Geometry: final body of the model. Coordinates: model frame, mm. Give positions to 0.01 mm unless a question says otherwise; leave off trailing zeros. Write each loop counter-clockwise with the first axis right and the second up, starting at its lowest first coordinate (ties: lowest second). Pieces come first, ordered by that corner, then holes.
from build123d import *

# Parameters (mm, degrees)
SKETCH1_W               = 127
SKETCH1_H               = 152.4
BOSS_EXTRUDE1_DEPTH     = 1.6
CHAMFER1_SIZE           = 5
CHAMFER2_SIZE           = 1.27
SKETCH4_OUTSIDE_W       = 168.678
SKETCH4_OUTSIDE_H       = 194.078
SKETCH4_OUTSIDE_W_2     = 146.645454771
SKETCH4_OUTSIDE_H_2     = 144.4
CUT_EXTRUDE3_DEPTH      = 0.0001
CUT_EXTRUDE4_DEPTH      = 100.203074549
CUT_EXTRUDE4_DEPTH_BACK = 100.203074549
SKETCH7_W               = 10
SKETCH7_H               = 16
CUT_EXTRUDE7_DEPTH      = 10
CUT_EXTRUDE8_REACH      = 101.203
SKETCH9_R               = 1.75


with BuildPart() as part:
    # Sketch1 → Boss-Extrude1 (new body)
    with BuildSketch(Plane(origin=(0, 0, 0), x_dir=(1, 0, 0), z_dir=(0, 1, 0))):
        Rectangle(SKETCH1_W, SKETCH1_H)
    extrude(amount=BOSS_EXTRUDE1_DEPTH)

    # Chamfer1
    chamfer1_edges = [part.edges().sort_by_distance(p)[0] for p in [
        (-63.5, 0.8, 76.2),
        (-63.5, 0.8, -76.2),
    ]]
    chamfer(chamfer1_edges, length=CHAMFER1_SIZE)

    # Chamfer2
    chamfer2_edges = [part.edges().sort_by_distance(p)[0] for p in [
        (63.5, 0.8, 76.2),
        (63.5, 0.8, -76.2),
    ]]
    chamfer(chamfer2_edges, length=CHAMFER2_SIZE)

    # Sketch4 outside → Cut-Extrude3 (cut)
    with BuildSketch(Plane(origin=(0, 1.6, 0), x_dir=(-1, 0, 0), z_dir=(0, 1, 0))):
        Rectangle(SKETCH4_OUTSIDE_W, SKETCH4_OUTSIDE_H)
        with Locations((0.842207065, 0)):
            Rectangle(SKETCH4_OUTSIDE_W_2, SKETCH4_OUTSIDE_H_2, mode=Mode.SUBTRACT)
    extrude(amount=-CUT_EXTRUDE3_DEPTH, mode=Mode.SUBTRACT)

    # Sketch5 → Cut-Extrude4 (cut, two sides: drawn at the far end of the back side and taken through both)
    with BuildSketch(Plane(origin=(0, 1.6, 0), x_dir=(1, 0, 0), z_dir=(0, 1, 0)).offset(-CUT_EXTRUDE4_DEPTH_BACK)):
        Polygon((-8.552407118, -467.338817365), (-53, -76.2), (-63.5, 16.2), (-107.947592882, 407.338817365), (-890.225227612, 318.4436316), (-790.830041847, -556.23400313), align=None)
    extrude(amount=CUT_EXTRUDE4_DEPTH + CUT_EXTRUDE4_DEPTH_BACK, mode=Mode.SUBTRACT)

    # Sketch7 → Cut-Extrude7 (cut)
    with BuildSketch(Plane(origin=(0, 1.6, 0), x_dir=(1, 0, 0), z_dir=(0, 1, 0))):
        with Locations((58.5, -68.2)):
            Rectangle(SKETCH7_W, SKETCH7_H)
    extrude(amount=-CUT_EXTRUDE7_DEPTH, mode=Mode.SUBTRACT)

    # Sketch9 → Cut-Extrude8 (cut, up to next)
    with BuildSketch(Plane(origin=(0, 1.6, 0), x_dir=(1, 0, 0), z_dir=(0, 1, 0)), mode=Mode.PRIVATE) as cut_extrude8_sk1:
        with Locations(Location((-43.7, 70.2, 0), (0, 0, 270))):
            Circle(SKETCH9_R)
    cut_extrude8_tool1 = extrude(cut_extrude8_sk1.sketch, amount=-CUT_EXTRUDE8_REACH, mode=Mode.PRIVATE) & part.part
    # Sketch9 → Cut-Extrude8 (cut, up to next)
    with BuildSketch(Plane(origin=(0, 1.6, 0), x_dir=(1, 0, 0), z_dir=(0, 1, 0)), mode=Mode.PRIVATE) as cut_extrude8_sk2:
        with Locations(Location((8.3, 70.2, 0), (0, 0, 270))):
            Circle(SKETCH9_R)
    cut_extrude8_tool2 = extrude(cut_extrude8_sk2.sketch, amount=-CUT_EXTRUDE8_REACH, mode=Mode.PRIVATE) & part.part
    # Sketch9 → Cut-Extrude8 (cut, up to next)
    with BuildSketch(Plane(origin=(0, 1.6, 0), x_dir=(1, 0, 0), z_dir=(0, 1, 0)), mode=Mode.PRIVATE) as cut_extrude8_sk3:
        with Locations(Location((30.252, -70.2, 0), (0, 0, 270))):
            Circle(SKETCH9_R)
    cut_extrude8_tool3 = extrude(cut_extrude8_sk3.sketch, amount=-CUT_EXTRUDE8_REACH, mode=Mode.PRIVATE) & part.part
    # Sketch9 → Cut-Extrude8 (cut, up to next)
    with BuildSketch(Plane(origin=(0, 1.6, 0), x_dir=(1, 0, 0), z_dir=(0, 1, 0)), mode=Mode.PRIVATE) as cut_extrude8_sk4:
        with Locations(Location((-39.188, -70.2, 0), (0, 0, 270))):
            Circle(SKETCH9_R)
    cut_extrude8_tool4 = extrude(cut_extrude8_sk4.sketch, amount=-CUT_EXTRUDE8_REACH, mode=Mode.PRIVATE) & part.part
    add(cut_extrude8_tool1.solids().sort_by_distance((-43.7, 1.6, -70.2))[0], mode=Mode.SUBTRACT)
    add(cut_extrude8_tool2.solids().sort_by_distance((8.3, 1.6, -70.2))[0], mode=Mode.SUBTRACT)
    add(cut_extrude8_tool3.solids().sort_by_distance((30.252, 1.6, 70.2))[0], mode=Mode.SUBTRACT)
    add(cut_extrude8_tool4.solids().sort_by_distance((-39.188, 1.6, 70.2))[0], mode=Mode.SUBTRACT)


solid = part.part
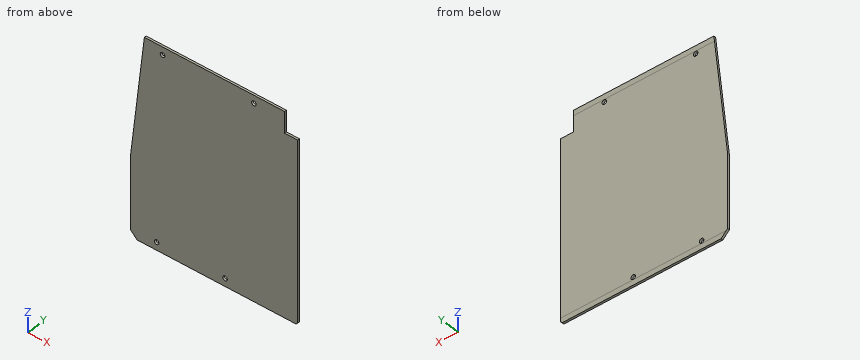
Q1. Section B-B on z = 70.2. Output: boundary loops of the cut face in (x, y).
Filled sheet:
outline: (-53.68, 0) - (-40.94, 0) - (-40.94, 1.6) - (-53.68, 1.6) - close; (-37.44, 0) - (28.5, 0) - (28.5, 1.6) - (-37.44, 1.6) - close; (32, 0) - (53.5, 0) - (53.5, 1.6) - (32, 1.6) - close
Q2. Section D-D on z = 33. Output: boundary loops of the cut face in (x, y).
Filled sheet:
outline: (-57.91, 0) - (63.5, 0) - (63.5, 1.6) - (-57.91, 1.6) - close
Q3. Section C-C on y = 1. Output: boundary loops of the cut face in (x, z).
Filled sheet:
outline: (-63.5, -71.2) - (-58.5, -76.2) - (62.23, -76.2) - (63.5, -74.93) - (63.5, 60.2) - (53.5, 60.2) - (53.5, 76.2) - (-53, 76.2) - (-63.5, -16.2) - close; hole circle Ø3.5 at (-43.7, -70.2); hole circle Ø3.5 at (-39.19, 70.2); hole circle Ø3.5 at (8.3, -70.2); hole circle Ø3.5 at (30.25, 70.2)
Q4. Ray query, line 1 along X through (y, z) = (1.15, -70.2); line 2 along Z through (x, y) = (31.5, 0.45); line 3 along X through (y, z) = (0.2, -8.5) (3 decimals). Return the intervals inside material, ascending.
Filled sheet:
line 1: x = -63.5 to -45.45, -41.95 to 6.55, 10.05 to 63.5
line 2: z = -76.2 to 68.97, 71.43 to 76.2
line 3: x = -62.625 to 63.5
